Design review of the part built by this model. Coordinates are the model's own, in mm. Coordinates: 2 decimals unless noted, no trailing zeros. Order: outer loops, then holes, each group sorted by start corner. A loop starts at its lowest first (then second) coordinate and runs counter-clockwise, first axis right, second up. Notation, with made-up numbers: M 21,50.5 L 66,50.5 A18 cw 66,84.5 Z; hole C 21.5,-11.75 d7. An arc over 180 degrees is marked long. Answer in a Markdown table with one row per item.
from build123d import *

# Parameters (mm, degrees)
SKETCH2_W           = 37.4
SKETCH2_H           = 85.5
BOSS_EXTRUDE1_DEPTH = 5.8
SKETCH3_W           = 12.7
SKETCH3_H           = 81.9
BOSS_EXTRUDE2_DEPTH = 4.7
SKETCH4_R           = 2.25
CUT_EXTRUDE1_DEPTH  = 5.8


with BuildPart() as part:
    # Sketch2 → Boss-Extrude1 (new body)
    with BuildSketch(Plane.XY):
        with Locations((18.7, 42.75)):
            Rectangle(SKETCH2_W, SKETCH2_H)
    extrude(amount=BOSS_EXTRUDE1_DEPTH)

    # Sketch3 → Boss-Extrude2 (add)
    with BuildSketch(Plane.XY.offset(5.8)):
        with Locations((18.7, 40.95)):
            Rectangle(SKETCH3_W, SKETCH3_H)
    extrude(amount=BOSS_EXTRUDE2_DEPTH)

    # Sketch4 → Cut-Extrude1 (cut)
    with BuildSketch(Plane(origin=(0, 0, 0), x_dir=(-1, 0, 0), z_dir=(0, 0, -1))):
        with Locations((-27.8, 78)):
            Circle(SKETCH4_R)
        with Locations((-9.6, 78)):
            Circle(SKETCH4_R)
        with Locations((-9.6, 8)):
            Circle(SKETCH4_R)
        with Locations((-27.8, 8)):
            Circle(SKETCH4_R)
    extrude(amount=-CUT_EXTRUDE1_DEPTH, mode=Mode.SUBTRACT)


solid = part.part
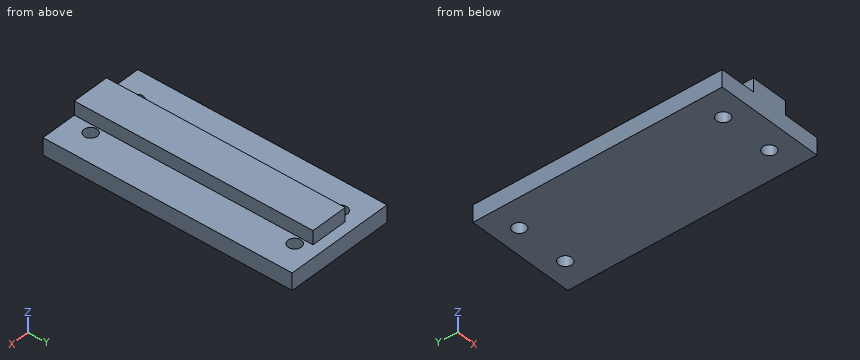
(1) Add section C-C, the plane z = 2.75. Give the boundary of the cut face in (x, y).
Return value:
| item | result |
|---|---|
| outline | M 0,0 L 37.4,0 L 37.4,85.5 L 0,85.5 Z; hole C 9.6,8 d4.5; hole C 9.6,78 d4.5; hole C 27.8,8 d4.5; hole C 27.8,78 d4.5 |
(2) Add section A-A, the plane x = 9.6. Give the boundary of the cut face in (y, z), and give its area (3 significant figures).
Return value:
| item | result |
|---|---|
| outline | M 0,0 L 5.75,0 L 5.75,5.8 L 0,5.8 Z; M 10.25,0 L 75.75,0 L 75.75,5.8 L 10.25,5.8 Z; M 80.25,0 L 85.5,0 L 85.5,5.8 L 80.25,5.8 Z |
| area | 444 mm2 |
(3) Add section B-B, the plane y = 8. Give the boundary of the cut face in (x, z), and give its area (3 significant figures).
Return value:
| item | result |
|---|---|
| outline | M 0,0 L 7.35,0 L 7.35,5.8 L 0,5.8 Z; M 11.85,0 L 25.55,0 L 25.55,5.8 L 25.05,5.8 L 25.05,10.5 L 12.35,10.5 L 12.35,5.8 L 11.85,5.8 Z; M 30.05,0 L 37.4,0 L 37.4,5.8 L 30.05,5.8 Z |
| area | 224 mm2 |
(4) Insertion check: pin 1 Ø4 at (x, z) = (16, 8.5) entering from +Y; pin 2 Ø4 at (y, z) = (27, 8.5) entering from -X. Each pin has a flat end and moves straight along its axis. Give the tip position at first contact, or say it passes through.
Return value:
| item | result |
|---|---|
| pin 1 | stops at y = 81.9 |
| pin 2 | stops at x = 12.35 |
(5) For line 1 along Y through (x, z) = (27.8, 1.9); line 2 along X through (y, z) = (79, 1.75); line 3 along X through (y, z) = (30, 7), list the stretches that pass through material, from the lowest coordinate up. Write a range as from..to.
Return value:
| item | result |
|---|---|
| line 1 | y = 0..5.75, 10.25..75.75, 80.25..85.5 |
| line 2 | x = 0..7.58, 11.62..25.78, 29.82..37.4 |
| line 3 | x = 12.35..25.05 |
(6) Add section D-D, the plane x = 14. Give the boundary of the cut face in (y, z), and give its area (3 significant figures).
Return value:
| item | result |
|---|---|
| outline | M 0,0 L 85.5,0 L 85.5,5.8 L 81.9,5.8 L 81.9,10.5 L 0,10.5 Z |
| area | 881 mm2 |
